```python
from build123d import *

# Parameters (mm, degrees)
CHAMFER1_SIZE = 0.762


with BuildPart() as part:
    # Sketch1 → Revolve1 (revolve)
    with BuildSketch(Plane.XY):
        Polygon((8.73125, 0), (11.1125, 0), (11.1125, 6.096), (6.35, 6.096), (6.35, -6.604), (8.73125, -6.604), align=None)
    revolve(axis=Axis((0, 0, 0), (0, -1, 0)))

    # Chamfer1
    chamfer1_edges = [part.edges().sort_by_distance(p)[0] for p in [
        (-6.35, 6.096, 0),
    ]]
    chamfer(chamfer1_edges, length=CHAMFER1_SIZE)


solid = part.part
```
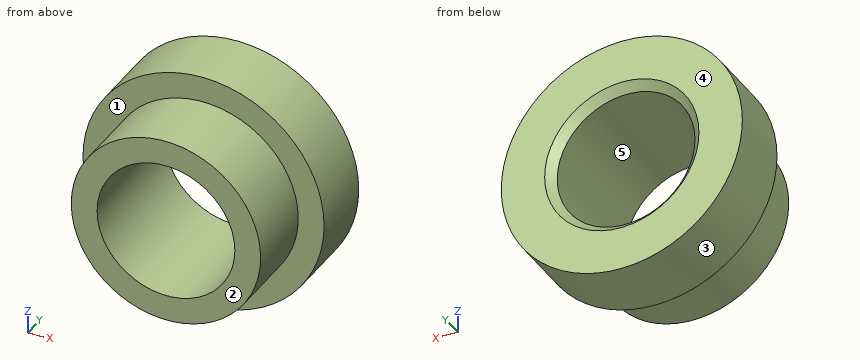
Geometry check sheet. Reference: the model listing, model coordinates, mm. Face numbers are marked on the shaded views. A direction names the side the tool comes from. Round coordinates to 2 decimals unless told otherwise and drop trailing zeros. Write each loop counter-clockwise with the first axis right and the second up, starting at its lowest first coordinate (ties: lowest second). Pieces come first, ordered by that corner, then holes. Notation, with made-up numbers: (4, -30.75) -> (16, -30.75) arc R33 cw to (16, 3.25) -> close; hole circle Ø11 at (34.5, 35). An arc over 180 degrees is marked (long way). Put each result on its own line as item: value.
1) Depth check by flat-ended pin: P1, Ø6, axis at x = 5.5, y = 1, coming from the +Z side; P2, Ø1.5, axis at y = -0.5, z = -1.5, coming from the -X side; P3, Ø6, axis at y = -1.5, z = -8, coming from the -X side; P4, Ø11.5, axis at x = 0, z = 0, coming from the -Y side. Enter the tip coordinate at first touch or a pass-through.
Recorded:
P1: stops at z = 10.83
P2: stops at x = -11.07
P3: stops at x = -9.71
P4: passes through
2) Cross-section at D-D, the plane x = 9.5. Enter the section's corners in (y, z).
Recorded:
outline: (0, -5.77) -> (6.1, -5.77) -> (6.1, 5.77) -> (0, 5.77) -> close
3) Cross-section at A-A, the plane z = 0. Enter the section's corners in (x, y).
Recorded:
outline: (-11.11, 0) -> (-8.73, 0) -> (-8.73, -6.6) -> (-6.35, -6.6) -> (-6.35, 5.33) -> (-7.11, 6.1) -> (-11.11, 6.1) -> close; (6.35, -6.6) -> (8.73, -6.6) -> (8.73, 0) -> (11.11, 0) -> (11.11, 6.1) -> (7.11, 6.1) -> (6.35, 5.33) -> close
4) Cross-section at C-C, the plane y = -1.5. Enter the section's corners in (x, z), plus the area to 3 significant figures.
Recorded:
outline: circle Ø17.46 at (0, 0); hole circle Ø12.7 at (0, 0)
area: 113 mm2
5) Access from +Z, -Z, +X, -X, +Y, -Y to the whole of each face (thin tool, end or side, straight path). Record for the marked faces 1 and 2.
Recorded:
face 1: -Y
face 2: +Z, -Z, +X, -X, -Y
6) Cross-section at B-B, the plane x = 0. Enter the section's corners in (y, z).
Recorded:
outline: (-6.6, -8.73) -> (0, -8.73) -> (0, -11.11) -> (6.1, -11.11) -> (6.1, -7.11) -> (5.33, -6.35) -> (-6.6, -6.35) -> close; (-6.6, 6.35) -> (5.33, 6.35) -> (6.1, 7.11) -> (6.1, 11.11) -> (0, 11.11) -> (0, 8.73) -> (-6.6, 8.73) -> close
7) Release check for a two-part mould opening along Z. For the marked faces 3, 4 and 5 record: pulls with the +Z half, pulls with the -Z half, needs draft (parallel to the pull), parting line crosses it, or undercut.
Recorded:
face 3: parting line crosses it
face 4: needs draft
face 5: undercut
8) Thickness scan on probe 1 along Z at (x, y) = (0, 2); probe 2 along Z at (x, y) = (0, -1.75); probe 3 along Y at (x, z) = (4.75, 9). Record the ranges inside material, lowest first. Write a range as from..to.
Recorded:
probe 1: z = -11.11..-6.35, 6.35..11.11
probe 2: z = -8.73..-6.35, 6.35..8.73
probe 3: y = 0..6.1
